```python
from build123d import *

# Parameters (mm, degrees)
SKETCH1_R            = 58.990480392
SKETCH1_R_2          = 51.253664764
BOSS_EXTRUDE4_DEPTH  = 3.81
BOSS_EXTRUDE8_DEPTH  = 6.35
BOSS_EXTRUDE11_DEPTH = 6.35
BOSS_EXTRUDE12_DEPTH = 1.27
BOSS_EXTRUDE13_DEPTH = 3.81
SKETCH1_10_R         = 71.690480392
BOSS_EXTRUDE14_DEPTH = 3.81


with BuildPart() as part:
    # Sketch1 → Boss-Extrude4 (new body)
    with BuildSketch(Plane.XY):
        with Locations(Location((0, 0, 0), (0, 0, 180))):
            Circle(SKETCH1_R)
        with Locations(Location((0, 0, 0), (0, 0, 180))):
            Circle(SKETCH1_R_2, mode=Mode.SUBTRACT)
    extrude(amount=BOSS_EXTRUDE4_DEPTH)

    # Sketch1_5 → Boss-Extrude8 (add)
    with BuildSketch(Plane.XY):
        with BuildLine():
            ThreePointArc((-16.590293497, 48.494332797), (-23.601953109, 45.495999397), (-30.091128704, 41.490506444))
            Line((-30.091128704, 41.490506444), (-8.151129624, 0))
            Line((-8.151129624, 0), (9.315576713, 0))
            Line((9.315576713, 0), (34.03630553, 38.320595736))
            ThreePointArc((34.03630553, 38.320595736), (26.945123943, 43.599294116), (19.052344379, 47.580944982))
            Line((19.052344379, 47.580944982), (-0.226270451, 13.588304137))
            Line((-0.226270451, 13.588304137), (-16.590293497, 48.494332797))
        make_face()
    extrude(amount=BOSS_EXTRUDE8_DEPTH)

    # Sketch1_7 → Boss-Extrude11 (add)
    with BuildSketch(Plane.XY):
        with BuildLine():
            Line((-16.590293497, -31.001033422), (-44.203304283, 25.942359996))
            ThreePointArc((-44.203304283, 25.942359996), (-47.205808206, 19.963712664), (-49.403992946, 13.644912337))
            Line((-49.403992946, 13.644912337), (-19.878887571, -47.24159164))
            ThreePointArc((-19.878887571, -47.24159164), (-14.115327494, -49.271651905), (-8.151129624, -50.601356084))
            Line((-8.151129624, -50.601356084), (0.554492374, -16.020255387))
            Line((0.554492374, -16.020255387), (6.439988792, -50.847464992))
            ThreePointArc((6.439988792, -50.847464992), (11.267949041, -49.99971476), (15.99284446, -48.694630893))
            Line((15.99284446, -48.694630893), (50.311661027, 9.781355549))
            ThreePointArc((50.311661027, 9.781355549), (48.850499882, 15.510216406), (46.739319117, 21.032693603))
            Line((46.739319117, 21.032693603), (15.784668638, -30.877460179))
            Line((15.784668638, -30.877460179), (9.315576713, -4.424898939))
            Line((9.315576713, -4.424898939), (-8.151129624, -4.424898939))
            Line((-8.151129624, -4.424898939), (-16.590293497, -31.001033422))
        make_face()
    extrude(amount=BOSS_EXTRUDE11_DEPTH)

    # Sketch1_8 → Boss-Extrude12 (add)
    with BuildSketch(Plane.XY):
        with BuildLine():
            ThreePointArc((-16.590293497, 48.494332797), (-23.601953109, 45.495999397), (-30.091128704, 41.490506444))
            Line((-30.091128704, 41.490506444), (-8.151129624, 0))
            Line((-8.151129624, 0), (9.315576713, 0))
            Line((9.315576713, 0), (34.03630553, 38.320595736))
            ThreePointArc((34.03630553, 38.320595736), (26.945123943, 43.599294116), (19.052344379, 47.580944982))
            Line((19.052344379, 47.580944982), (-0.226270451, 13.588304137))
            Line((-0.226270451, 13.588304137), (-16.590293497, 48.494332797))
        make_face()
    extrude(amount=BOSS_EXTRUDE12_DEPTH)

    # Sketch1_9 → Boss-Extrude13 (add)
    with BuildSketch(Plane.XY):
        with BuildLine():
            Line((-16.590293497, -31.001033422), (-44.203304283, 25.942359996))
            ThreePointArc((-44.203304283, 25.942359996), (-47.205808206, 19.963712664), (-49.403992946, 13.644912337))
            Line((-49.403992946, 13.644912337), (-19.878887571, -47.24159164))
            ThreePointArc((-19.878887571, -47.24159164), (-14.115327494, -49.271651905), (-8.151129624, -50.601356084))
            Line((-8.151129624, -50.601356084), (0.554492374, -16.020255387))
            Line((0.554492374, -16.020255387), (6.439988792, -50.847464992))
            ThreePointArc((6.439988792, -50.847464992), (11.267949041, -49.99971476), (15.99284446, -48.694630893))
            Line((15.99284446, -48.694630893), (50.311661027, 9.781355549))
            ThreePointArc((50.311661027, 9.781355549), (48.850499882, 15.510216406), (46.739319117, 21.032693603))
            Line((46.739319117, 21.032693603), (15.784668638, -30.877460179))
            Line((15.784668638, -30.877460179), (9.315576713, -4.424898939))
            Line((9.315576713, -4.424898939), (-8.151129624, -4.424898939))
            Line((-8.151129624, -4.424898939), (-16.590293497, -31.001033422))
        make_face()
        with BuildLine():
            ThreePointArc((-16.590293497, 48.494332797), (-23.601953109, 45.495999397), (-30.091128704, 41.490506444))
            Line((-30.091128704, 41.490506444), (-8.151129624, 0))
            Line((-8.151129624, 0), (9.315576713, 0))
            Line((9.315576713, 0), (34.03630553, 38.320595736))
            ThreePointArc((34.03630553, 38.320595736), (26.945123943, 43.599294116), (19.052344379, 47.580944982))
            Line((19.052344379, 47.580944982), (-0.226270451, 13.588304137))
            Line((-0.226270451, 13.588304137), (-16.590293497, 48.494332797))
        make_face()
    extrude(amount=BOSS_EXTRUDE13_DEPTH)

    # Sketch1_10 → Boss-Extrude14 (add)
    with BuildSketch(Plane.XY):
        with Locations(Location((0, 0, 0), (0, 0, 180))):
            Circle(SKETCH1_10_R)
    extrude(amount=BOSS_EXTRUDE14_DEPTH)


solid = part.part
```
Verification items for the finished model (mm, model axes). A direction names the side the tool comes from. Round coordinates to 2 decimals unless told otherwise and drop trailing zeros. Write each loop counter-clockwise with the first axis right and the second up, starting at its lowest first coordinate (ties: lowest second). Pieces come first, ordered by that corner, then holes. Notation, with made-up numbers: (-8.5, -38.75) - (0.5, -38.75) arc R23 cw to (0.5, -25.75) - close; hole circle Ø3 at (73, -13.5). An arc over 180 degrees is marked (long way). Answer as a JSON object with one key per item and string values. Group by question number.
Q1. Section check D-D, the plane x = 43. Enter the section's corners in (y, z).
Q2. Section check A-A, the plane y = -42. Enter the section's corners in (x, z).
Q3. Mould release check, pull along Y, two halves, no side actions. Record for faces 5 (the cylindrical face through (-23.507, 45.545, 5.062)), 6 (the flat face through (-3, -21, 6.35)), 7 (the flat face through (-19.275, 21.036, 5.062)): released by +Y, released by -Y, zero draft, split by the parting line, or undercut.
Q4. Thickness scan on line 1 (Z direction, x = -34, y = 29); line 2 (X direction, y = 1.5, z = 2.5); line 3 (X direction, y = -22.5, z = 5.5). Record the ranges inside material, lowest first.
Q5. Go/stop test with flat-tipped pins: pin 1 Ø2 at (x, z) = (45.5, 5) entering from -Y; pin 2 Ø8 at (x, y) = (25, 13.5) entering from +Z; pin 3 Ø1.3 at (x, z) = (-1, 5.5) entering from +Y. Record where each tip stops, or that it passes through.
Q6. Section check C-C, the plane z = 2.25. Enter the section's corners in (x, y), plus the area to 3 significant figures.
Q7. Section check B-B, the plane x = -33.5. Enter the section's corners in (y, z).
Q8. Tool access check on faces 1 (the cylindrical face through (48.875, 15.431, 5.062)), 2 (the flat face through (32.91, -19.87, 5.06)), 3 (the flat face through (-3.86, -33.55, 5.06)), 4 (the flat face through (-30.204, -2.928, 5.062)). Record the directions out of +Z, -Z, +X, -X, +Y, -Y that give a thin tool (end or side, any length) a straight path to the whole face; none if there is none.
Found:
{
 "1": {"outline": "(-57.36, 0) - (57.36, 0) - (57.36, 3.81) - (14.76, 3.81) - (14.76, 6.35) - (-2.68, 6.35) - (-2.68, 3.81) - (-57.36, 3.81) - close"},
 "2": {"outline": "(-58.1, 0) - (58.1, 0) - (58.1, 3.81) - (19.92, 3.81) - (19.92, 6.35) - (4.94, 6.35) - (4.94, 3.81) - (-5.99, 3.81) - (-5.99, 6.35) - (-22.42, 6.35) - (-22.42, 3.81) - (-58.1, 3.81) - close"},
 "3": {"face 5": "released by +Y", "face 6": "zero draft", "face 7": "undercut"},
 "4": {"line 1": "z = 0 to 3.81", "line 2": "x = -71.67 to 71.67", "line 3": "x = -31.88 to -20.71, -13.89 to -1.08, 1.65 to 13.74, 20.78 to 31.37"},
 "5": {"pin 1": "stops at y = -0.12", "pin 2": "stops at z = 3.81", "pin 3": "stops at y = 16.63"},
 "6": {"outline": "circle Ø143.38 at (0, 0)", "area": "16,100 mm^2"},
 "7": {"outline": "(-63.38, 0) - (63.38, 0) - (63.38, 3.81) - (3.87, 3.81) - (3.87, 6.35) - (-19.15, 6.35) - (-19.15, 3.81) - (-63.38, 3.81) - close"},
 "8": {"face 1": "+Z, +X, +Y", "face 2": "+Z, +X, -Y", "face 3": "+Z, -Y", "face 4": "+Z"}
}
